Can you work these out from the model? Positions are in its coordinate system, mm. A direction names the side the tool comes from. Coordinates: 2 decimals unless noted, no trailing zeros. Write each loop counter-clockwise with the first axis right and the second up, starting at its lowest first coordinate (ties: lowest second). Pieces come first, ordered by that corner, then holes. Notation, with made-up numbers: (-32, -3.5) -> (10, -3.5) arc R7 ccw to (10, 9.5) -> close; hole circle Ø6 at (-5.75, -20). An arc over 180 degrees is marked (long way). Answer as CSV lines item,"result". Start each with the question number.
```python
from build123d import *

# Parameters (mm, degrees)
SKETCH1_W           = 12.7
SKETCH1_H           = 101.6
BOSS_EXTRUDE1_DEPTH = 19.05
FILLET2_RADIUS      = 6.35
FILLET2_LENGTH      = 38.1
SKETCH2_R           = 3.81
CUT_EXTRUDE1_DEPTH  = 38.1
FILLET3_RADIUS      = 6.35
FILLET3_LENGTH      = 38.1
SKETCH3_W           = 25.4
SKETCH3_H           = 25.4
CUT_EXTRUDE2_DEPTH  = 56.72102386
FILLET4_RADIUS      = 6.35
FILLET4_LENGTH      = 25.4
SKETCH4_W           = 45.439126892
SKETCH4_H           = 74.581358872
CUT_EXTRUDE3_DEPTH  = 56.72102386
SKETCH5_R           = 5.08
BOSS_EXTRUDE2_DEPTH = 50.8


with BuildPart() as part:
    # Sketch1 → Boss-Extrude1 (new, symmetric)
    with BuildSketch(Plane.XY):
        Rectangle(SKETCH1_W, SKETCH1_H)
    extrude(amount=BOSS_EXTRUDE1_DEPTH, both=True)

    # Fillet2: full round fillet: the end face becomes a half cylinder, R = half its width
    fillet2_face = Plane((0, -50.8, 0), x_dir=(0, 0, 1), z_dir=(0, -1, 0))  # on the end face: x along it, z out of the body
    fillet2_slab = fillet2_face.offset(-FILLET2_RADIUS / 2) * Box(FILLET2_LENGTH, 2 * FILLET2_RADIUS, FILLET2_RADIUS, mode=Mode.PRIVATE)  # the body's end, R deep
    fillet2_round = Plane((0, -44.45, 0), x_dir=(0, -1, 0), z_dir=(0, 0, 1)) * Cylinder(FILLET2_RADIUS, FILLET2_LENGTH, mode=Mode.PRIVATE)  # its axis R under the face
    add(fillet2_slab - fillet2_round, mode=Mode.SUBTRACT)

    # Sketch2 → Cut-Extrude1 (cut)
    with BuildSketch(Plane.XY.offset(19.05)):
        with Locations((0, -44.45)):
            Circle(SKETCH2_R)
    cut_extrude1 = extrude(amount=-CUT_EXTRUDE1_DEPTH, mode=Mode.SUBTRACT)

    # Mirror3: Cut-Extrude1 across plane
    add(cut_extrude1.mirror(Plane.ZX), mode=Mode.SUBTRACT)

    # Fillet3: full round fillet: the end face becomes a half cylinder, R = half its width
    fillet3_face = Plane((0, 50.8, 0), x_dir=(0, 0, 1), z_dir=(0, 1, 0))  # on the end face: x along it, z out of the body
    fillet3_slab = fillet3_face.offset(-FILLET3_RADIUS / 2) * Box(FILLET3_LENGTH, 2 * FILLET3_RADIUS, FILLET3_RADIUS, mode=Mode.PRIVATE)  # the body's end, R deep
    fillet3_round = Plane((0, 44.45, 0), x_dir=(0, 1, 0), z_dir=(0, 0, 1)) * Cylinder(FILLET3_RADIUS, FILLET3_LENGTH, mode=Mode.PRIVATE)  # its axis R under the face
    add(fillet3_slab - fillet3_round, mode=Mode.SUBTRACT)

    # Sketch3 → Cut-Extrude2 (cut, through all)
    with BuildSketch(Plane.ZY.offset(6.35)):
        with Locations((0, 38.1)):
            Rectangle(SKETCH3_W, SKETCH3_H)
    extrude(amount=-CUT_EXTRUDE2_DEPTH, mode=Mode.SUBTRACT)

    # Fillet4: full round fillet: the end face becomes a half cylinder, R = half its width
    fillet4_face = Plane((0, 25.4, 0), x_dir=(0, 0, -1), z_dir=(0, 1, 0))  # on the end face: x along it, z out of the body
    fillet4_slab = fillet4_face.offset(-FILLET4_RADIUS / 2) * Box(FILLET4_LENGTH, 2 * FILLET4_RADIUS, FILLET4_RADIUS, mode=Mode.PRIVATE)  # the body's end, R deep
    fillet4_round = Plane((0, 19.05, 0), x_dir=(0, 1, 0), z_dir=(0, 0, -1)) * Cylinder(FILLET4_RADIUS, FILLET4_LENGTH, mode=Mode.PRIVATE)  # its axis R under the face
    add(fillet4_slab - fillet4_round, mode=Mode.SUBTRACT)

    # Sketch4 → Cut-Extrude3 (cut, through all)
    with BuildSketch(Plane(origin=(6.35, 0, 0), x_dir=(0, 0, -1), z_dir=(1, 0, 0))):
        with Locations((3.669563446, -18.240679436)):
            Rectangle(SKETCH4_W, SKETCH4_H)
    extrude(amount=-CUT_EXTRUDE3_DEPTH, mode=Mode.SUBTRACT)

    # Sketch5 → Boss-Extrude2 (add)
    with BuildSketch(Plane.XZ.offset(-19.05)):
        with Locations(Location((0, 0, 0), (0, 0, 180))):
            Circle(SKETCH5_R)
    extrude(amount=BOSS_EXTRUDE2_DEPTH)

    # Sketch8 → Revolve-Thin1 (revolve)
    with BuildSketch(Plane.XY):
        with BuildLine():
            ThreePointArc((10.16, -41.91), (7.184204897, -34.725795103), (0, -31.75))
            Line((0, -31.75), (0, -31.242))
            ThreePointArc((0, -31.242), (7.543415142, -34.366584858), (10.668, -41.91))
            Line((10.668, -41.91), (10.16, -41.91))
        make_face()
    revolve(axis=Axis((0, -58.668197781, 0), (0, 1, 0)))


solid = part.part
```
Q1. Imagine slicing it at B-B (x = 0). Write out the boundary of the cut face in (y, z).
Q2. Imagine slicing it at C-C (y = 5). Write out the boundary of the cut face in (x, z).
Q3. For pin 1 (8 mm diameter, centred on x = -1, y = -8.5, fed in from +Z); pin 2 (1 mm diameter, centred on x = 6.5, y = 4.5, fed in from -Z); pin 3 (3 mm diameter, centred on x = 1, z = 1, fed in from -Y); pin 4 (7 mm diameter, centred on y = 28, z = -17.5, fed in from -X), each with a flat end and sliding along its axis, tell me the tip position at first contact or that it passes through.
Q4. I need wall thicknesses on L1, parallel to X at y = 44.45, z = -14.25; L2, parallel to Y at x = 0.25, z = -14; L3, parallel to Z at x = 4.5, y = 31. Which ranges of each line are inside material? Lowest first, please.
Q5. If we mould it in two halves opening along Y, with no side actions, what happens to faces 1 (the face through (0, 35, 12.7)), 2 (the face through (0.1, 50.8, -15.8)), 3 (the face through (-3, 19.05, 5)), 4 (the face through (0.661, -5.994, -5.037))? For each: released by +Y, released by -Y, zero draft, split by the parting line, or undercut.
Q6. Imagine slicing it at A-A (z = 4). Write out the boundary of the cut face in (x, y).
Q7. Imagine slicing it at D-D (z = 0). Write out the boundary of the cut face in (x, y).
Q8. Which directions (+Z, -Z, +X, -X, +Y, -Y) give clear straight access to the entire face, cutting with the end or side of a thin tool? Please do faces 5 (the face through (0, 32, 19.05)), 6 (the face through (-0.1, 25.4, -0.2)).
Entries:
1,outline,"(-41.91, -10.67) arc R10.67 ccw to (-31.75, -3.25) -> (-31.75, -5.08) -> (19.05, -5.08) -> (19.05, -19.05) -> (40.64, -19.05) -> (40.64, -12.7) -> (25.4, -12.7) -> (25.4, 12.7) -> (40.64, 12.7) -> (40.64, 19.05) -> (19.05, 19.05) -> (19.05, 5.08) -> (-31.75, 5.08) -> (-31.75, 3.25) arc R10.67 ccw to (-41.91, 10.67) -> (-41.91, 10.16) arc R10.16 cw to (-41.91, -10.16) -> close; (48.26, -19.05) -> (50.8, -19.05) -> (50.8, -12.7) -> (48.26, -12.7) -> close; (48.26, 12.7) -> (50.8, 12.7) -> (50.8, 19.05) -> (48.26, 19.05) -> close"
2,outline,"circle Ø10.16 at (0, 0)"
3,pin 1,"z = 5.08"
3,pin 2,"through"
3,pin 3,"y = -32.18"
3,pin 4,"x = -6.35"
4,L1,"-6.35 to -3.81, 3.81 to 6.35"
4,L2,"19.05 to 40.65, 48.25 to 50.8"
4,L3,"-19.05 to -12.7, 12.7 to 19.05"
5,face 1,"zero draft"
5,face 2,"released by +Y"
5,face 3,"undercut"
5,face 4,"undercut"
6,outline,"(-9.89, -41.91) -> (-9.34, -41.91) arc R9.34 cw to (9.34, -41.91) -> (9.89, -41.91) arc R9.89 ccw to start; (-6.35, 19.05) -> (-3.13, 19.05) -> (-3.13, -31.75) -> (3.13, -31.75) -> (3.13, 19.05) -> (6.35, 19.05) arc R6.35 ccw to start"
7,outline,"(-10.67, -41.91) -> (-10.16, -41.91) arc R10.16 cw to (10.16, -41.91) -> (10.67, -41.91) arc R10.67 ccw to (3.25, -31.75) -> (5.08, -31.75) -> (5.08, 19.05) -> (6.35, 19.05) arc R6.35 ccw to (-6.35, 19.05) -> (-5.08, 19.05) -> (-5.08, -31.75) -> (-3.25, -31.75) arc R10.67 ccw to start"
8,face 5,"+Z, +X, -X, +Y, -Y"
8,face 6,"+Y"
